```python
from build123d import *

# Parameters (mm, degrees)
F0_W     = 389
F0_H     = 140
F0_R     = 5
F0_R_2   = 2.5
F1_DEPTH = 12
F2_R     = 2.5
F3_DEPTH = 25


with BuildPart() as f1:
    # F0 (on Front) → F1 (new body)
    with BuildSketch(Plane.XZ):
        Rectangle(F0_W, F0_H)
        with Locations((-134.5, -61)):
            Circle(F0_R, mode=Mode.SUBTRACT)
        with Locations((-188.5, -40)):
            Circle(F0_R_2, mode=Mode.SUBTRACT)
        with Locations((-152.5, -40)):
            Circle(F0_R_2, mode=Mode.SUBTRACT)
        with Locations((0, -61)):
            Circle(F0_R, mode=Mode.SUBTRACT)
        with Locations((134.5, -61)):
            Circle(F0_R, mode=Mode.SUBTRACT)
        with Locations((152.5, -40)):
            Circle(F0_R_2, mode=Mode.SUBTRACT)
        with Locations((188.5, -40)):
            Circle(F0_R_2, mode=Mode.SUBTRACT)
        with Locations((-188.5, 40)):
            Circle(F0_R_2, mode=Mode.SUBTRACT)
        with Locations((-152.5, 40)):
            Circle(F0_R_2, mode=Mode.SUBTRACT)
        with Locations((152.5, 40)):
            Circle(F0_R_2, mode=Mode.SUBTRACT)
        with Locations((188.5, 40)):
            Circle(F0_R_2, mode=Mode.SUBTRACT)
    extrude(amount=F1_DEPTH)

    # F2 (on face) → F3 (cut)
    with BuildSketch(Plane(origin=(0, 0, -70), x_dir=(1, 0, 0), z_dir=(0, 0, -1))):
        with Locations((0, 6)):
            Circle(F2_R)
        with Locations((134.5, 6)):
            Circle(F2_R)
        with Locations((-134.5, 6)):
            Circle(F2_R)
    extrude(amount=-F3_DEPTH, mode=Mode.SUBTRACT)


solid = f1.part
```
The listing builds one solid part. Answer for the finished solid, in the listing's coordinates (mm). Coordinates: 2 decimals unless noted, no trailing zeros. Return JSON: item names as keys, results as strings. Group by question number.
1. Straight lines are drawn through the part: L1, parallel to X at y = -6, z = -68.45; L2, parallel to Z at x = 135, y = -9.5; L3, parallel to Z at x = -138, y = -1.25. For each, find the intervals that lie inside material, in ascending order.
2. Determine the mould class of faces 1 (the flat face through (-3, -6, 70)), 2 (the cylindrical face through (3, -6, -57)), 3 (the flat face through (-194.5, -6, -1)) for opening direction X: released by +X, released by -X, zero draft, split by the parting line, or undercut.
3. Given pin 1 (6 mm diameter, centred on x = 152.5, z = 40, fed in from +Y); pin 2 (6 mm diameter, centred on x = 134.5, z = -61, fed in from -Y); pin 3 (4.5 mm diameter, centred on x = -134.5, y = -6, fed in from -Z), each flat-ended and moving along its own axis, determine where each tip first touches the part or whether it passes through.
Ans:
{
 "1": {"L1": "-194.5 to -137, -132 to -2.5, 2.5 to 132, 137 to 194.5", "L2": "-70 to -65.97, -56.03 to 70", "L3": "-70 to -64.57, -57.43 to 70"},
 "2": {"face 1": "zero draft", "face 2": "undercut", "face 3": "released by -X"},
 "3": {"pin 1": "y = 0", "pin 2": "through", "pin 3": "z = -45"}
}
